Geometry check sheet. Reference: the model listing, model coordinates, mm. A direction names the side the tool comes from. Give positions to 0.01 mm unless a question says otherwise; leave off trailing zeros. Write each loop counter-clockwise with the first axis right and the second up, starting at its lowest first coordinate (ties: lowest second). Pieces come first, ordered by that corner, then holes.
(1) Tool access check on faces 4 (the cylindrical face through (-0.956, 1.493, 0.907)), 5 (the flat face through (9, 1, 27)). Record the directions out of +Z, -Z, +X, -X, +Y, -Y that give a thin tool (end or side, any length) a straight path to the whole face; none if there is none.
(2) Cross-section at B-B (z = 26.99). Record the boundary of the cut face in (x, y).
(3) Thickness scan on line 1 along Z through (x, y) = (-65.6, 1.5); line 2 along Z through (x, y) = (-65.6, 0.75); line 3 along Z through (x, y) = (-51.5, 1.3). Record the ranges inside material, lowest first.
(4) Cross-section at C-C (z = 37). Record the boundary of the cut face in (x, y), and give its area (3 significant figures).
(5) Cross-section at D-D (x = -55). Record the boundary of the cut face in (y, z), and give its area (3 significant figures).
(6) Mould release check, pull along X, two halves, no side actions. Record for faces 1 (the cylindrical face through (-87.459, 1.014, 56.777)), 2 (the flat face through (0.2, 2, 24.8)), 3 (the flat face through (-42, 1, 27)): +X half, -X half, draft (parallel to the pull), parting line (faces both ways), or undercut.
(7) Depth check by flat-ended pin: P1, Ø1.5, axis at x = -3.5, z = 27.5, coming from the +Y side; P2, Ø4.5, axis at x = 4.5, z = 26.99, coming from the +Y side. Enter the tip coordinate at first touch or a pass-through.
(8) Cross-section at A-A (x = -65.6). Record the boundary of the cut face in (y, z).
Autodesk Inventor part; units mm, degrees
ref_plane "YZ Plane" through (0, 0, 0) normal (1, 0, 0) x (0, 1, 0)
ref_plane "XZ Plane" through (0, 0, 0) normal (0, 1, 0) x (-1, 0, 0)
ref_plane "XY Plane" through (0, 0, 0) normal (0, 0, 1) x (1, 0, 0)
sketch "Sketch1" plane through (0, 0, 0) normal (0, 1, 0) x (-1, 0, 0)
  line L0 (0, 0) -> (85.6, 0)
  line L1 (85.6, 0) -> (85.6, 53.98)
  line L2 (85.6, 53.98) -> (0, 53.98)
  line L3 (0, 53.98) -> (0, 0)
  line L4 (0, 53.98) -> (0, 50.8)
  line L5 (0, 50.8) -> (3.18, 50.8)
  circle A0 centre (3.18, 50.8) radius 3.18
  line L6 (85.6, 53.98) -> (85.6, 57.98)
  line L7 (85.6, 57.98) -> (0, 57.98)
  line L8 (0, 57.98) -> (-9, 57.98)
  line L9 (-9, 57.98) -> (-9, 0)
  line L10 (-9, 0) -> (0, 0)
  line L11 (0, 26.99) -> (-4.5, 26.99)
  circle A1 centre (-4.5, 26.99) radius 2.5
  line L12 (85.6, 55.98) -> (65.6, 55.98)
  circle A2 centre (65.6, 55.98) radius 1
  line L13 (0, 26.99) -> (85.6, 26.99)
  line L14 (85.6, -4) -> (0, -4)
  line L15 (0, -4) -> (-9, -4)
  circle A3 centre (65.6, -2) radius 1
  line L16 (85.6, -4) -> (85.6, 0)
  line L17 (-9, -4) -> (-9, 0)
  line L18 (85.6, 57.98) -> (88.6, 57.98)
  line L19 (88.6, 57.98) -> (88.6, -4)
  line L20 (88.6, -4) -> (85.6, -4)
  line L21 (85.6, -4) -> (85.6, 57.98)
  line L22 (85.6, 53.98) -> (88.6, 53.98)
  line L23 (85.6, 0) -> (88.6, 0)
  circle A4 centre (3.18, 3.18) radius 3.18
  point P0 (3.18, 0)
  point P1 (0, 3.18)
  point P2 (3.18, 53.98)
  dimension "d0" = 85.6
  dimension "d1" = 53.98
  dimension "d2" = 3.18
  dimension "d3" = 3.18
  dimension "d4" = 4
  dimension "d5" = 9
  dimension "d6" = 5
  dimension "d7" = 20
  dimension "d8" = 2
  dimension "d9" = 3
extrude "Extrusion1" add sketch "Sketch1" along normal blind 2 contours L3 A4 L0 | L10 L9 L8 L7 L6 L2 L3 | L0 L16 L14 L15 L17 L10 | L3 L2 A0 | L6 L18 L19 L22
extrude "Extrusion2" add sketch "Sketch1" along normal blind 1 contours A4 L3 L13 L1 L0 | A4 | L3 A0 L2 L1 L13 | A0
extrude "Extrusion3" add sketch "Sketch1" along normal blind 2 contours L23 L19 L20 L16
extrude "Extrusion4" add sketch "Sketch1" along normal blind 1.5 contours L1 L22 L19 L23
fillet "Fillet1" radius 24.13 1 edges at (-85.6, 1.5, 26.99)
fillet "Fillet2" radius 4 4 edges at (-88.6, 1, 57.98) (-88.6, 1, -4) (9, 1, -4) (9, 1, 57.98)
properties part number "magnet card bottom"
Reply:
1. face 4: +Y
1. face 5: +Z, -Z, +X, +Y, -Y
2. outline: (-88.6, 0) - (2, 0) - (2, 2) - (0, 2) - (0, 1) - (-85.6, 1) arc R24.13 ccw to (-88.6, 1.5) - close; (7, 0) - (9, 0) - (9, 2) - (7, 2) - close
3. line 1: z = -4 to -3, -1 to 0, 53.98 to 54.98, 56.98 to 57.98
3. line 2: z = -4 to -3, -1 to 54.98, 56.98 to 57.98
3. line 3: z = -4 to 0, 53.98 to 57.98
4. outline: (-88.6, 0) - (9, 0) - (9, 2) - (0, 2) - (0, 1) - (-85.6, 1) arc R24.13 ccw to (-88.6, 1.5) - close
4. area: 107 mm2
5. outline: (0, -4) - (2, -4) - (2, 0) - (1, 0) - (1, 53.98) - (2, 53.98) - (2, 57.98) - (0, 57.98) - close
5. area: 70.0 mm2
6. face 1: -X half
6. face 2: draft
6. face 3: undercut
7. P1: stops at y = 1
7. P2: passes through
8. outline: (0, -4) - (2, -4) - (2, -3) - (0, -3) - close; (0, -1) - (2, -1) - (2, 0) - (1, 0) - (1, 53.98) - (2, 53.98) - (2, 54.98) - (0, 54.98) - close; (0, 56.98) - (2, 56.98) - (2, 57.98) - (0, 57.98) - close
